```python
from build123d import *

# Parameters (mm, degrees)
SKETCH_1_W                = 42
SKETCH_1_H                = 42
SKETCH_1_R                = 1.85
EXTRUDE_1_DEPTH           = 8
FILLET_2_R                = 2
FILLET_3_R                = 2
FILLET_4_R                = 2
FILLET_5_R                = 2
SKETCH_2_W                = 6
SKETCH_2_H                = 10.5
SKETCH_2_W_2              = 4
SKETCH_2_H_2              = 26
SKETCH_2_W_3              = 13
SKETCH_2_H_3              = 5.5
CUT_EXTRUDE_1_DEPTH       = 6
SKETCH_3_W                = 5.557975162
SKETCH_3_H                = 9
CUT_EXTRUDE_2_DEPTH       = 3
CUT_EXTRUDE_3_DEPTH       = 31.757112998
CUT_EXTRUDE_13_DEPTH      = 31.757112998
SKETCH_6_W                = 14
SKETCH_6_H                = 11
CUT_EXTRUDE_4_DEPTH       = 31.757112998
CUT_EXTRUDE_5_DEPTH       = 3
HOLE_WIZARD_2_D           = 3.6
HOLE_WIZARD_2_DEPTH       = 8
HOLE_WIZARD_2_CSINK_D     = 6.6
HOLE_WIZARD_2_CSINK_ANGLE = 90


with BuildPart() as part:
    # 草图1 → 凸台-拉伸1 (new body)
    with BuildSketch(Plane(origin=(0, 0, 0), x_dir=(1, 0, 0), z_dir=(0, 1, 0))):
        Rectangle(SKETCH_1_W, SKETCH_1_H)
        with Locations(Location((15.5, 15.5, 0), (0, 0, 270))):
            Circle(SKETCH_1_R, mode=Mode.SUBTRACT)
        with Locations(Location((-15.5, 15.5, 0), (0, 0, 270))):
            Circle(SKETCH_1_R, mode=Mode.SUBTRACT)
        with Locations(Location((-15.5, -15.5, 0), (0, 0, 270))):
            Circle(SKETCH_1_R, mode=Mode.SUBTRACT)
        with Locations(Location((15.5, -15.5, 0), (0, 0, 270))):
            Circle(SKETCH_1_R, mode=Mode.SUBTRACT)
    extrude(amount=EXTRUDE_1_DEPTH)

    # 圆角2
    fillet_2_edges = [part.edges().sort_by_distance(p)[0] for p in [
        (-21, 4, -21),
    ]]
    fillet(fillet_2_edges, radius=FILLET_2_R)

    # 圆角3
    fillet_3_edges = [part.edges().sort_by_distance(p)[0] for p in [
        (-21, 4, 21),
    ]]
    fillet(fillet_3_edges, radius=FILLET_3_R)

    # 圆角4
    fillet_4_edges = [part.edges().sort_by_distance(p)[0] for p in [
        (21, 4, 21),
    ]]
    fillet(fillet_4_edges, radius=FILLET_4_R)

    # 圆角5
    fillet_5_edges = [part.edges().sort_by_distance(p)[0] for p in [
        (21, 4, -21),
    ]]
    fillet(fillet_5_edges, radius=FILLET_5_R)

    # 草图2 → 切除-拉伸1 (cut)
    with BuildSketch(Plane.XZ):
        with Locations((18, 7.7)):
            Rectangle(SKETCH_2_W, SKETCH_2_H)
        with Locations((-19, -0.23)):
            Rectangle(SKETCH_2_W_2, SKETCH_2_H_2)
        with Locations((14.5, -9.635)):
            Rectangle(SKETCH_2_W_3, SKETCH_2_H_3)
    extrude(amount=-CUT_EXTRUDE_1_DEPTH, mode=Mode.SUBTRACT)

    # 草图3 → 切除-拉伸2 (cut)
    with BuildSketch(Plane.XZ):
        with Locations((18.221012419, -3)):
            Rectangle(SKETCH_3_W, SKETCH_3_H)
    extrude(amount=-CUT_EXTRUDE_2_DEPTH, mode=Mode.SUBTRACT)

    # 草图5 → 切除-拉伸3 (cut, through all)
    with BuildSketch(Plane.XZ):
        Polygon((-15.5, -21), (-10, -15.5), (10, -15.5), (15.5, -21), align=None)
    extrude(amount=-CUT_EXTRUDE_3_DEPTH, mode=Mode.SUBTRACT)

    # 草图10 → 切除-拉伸13 (cut, through all)
    with BuildSketch(Plane(origin=(0, 8, 0), x_dir=(1, 0, 0), z_dir=(0, 1, 0))):
        with BuildLine():
            Line((7, -21.5), (2.5, -21.5))
            Line((2.5, -21.5), (2.5, -17))
            ThreePointArc((2.5, -17), (10.181980515, -13.818019485), (7, -21.5))
        make_face()
    extrude(amount=-CUT_EXTRUDE_13_DEPTH, mode=Mode.SUBTRACT)

    # 草图6 → 切除-拉伸4 (cut, through all)
    with BuildSketch(Plane.XZ):
        with Locations((-3, 15.5)):
            Rectangle(SKETCH_6_W, SKETCH_6_H)
    extrude(amount=-CUT_EXTRUDE_4_DEPTH, mode=Mode.SUBTRACT)

    # 草图7 → 切除-拉伸5 (cut)
    with BuildSketch(Plane.XZ):
        Polygon((-9.016278831, 15.5), (-15.5, 9.016278831), (-15.5, -9.016278831), (-9.016278831, -15.5), (9.016278831, -15.5), (15.5, -9.016278831), (15.5, 9.016278831), (9.016278831, 15.5), align=None)
    extrude(amount=-CUT_EXTRUDE_5_DEPTH, mode=Mode.SUBTRACT)

    # 打孔尺寸(%根据十字)槽半沉头木螺钉的类型2
    with Locations(Plane(origin=(0, 8, 0), x_dir=(1, 0, 0), z_dir=(0, 1, 0))):
        with Locations((15.5, -15.5), (-15.5, -15.5), (-15.5, 15.5), (15.5, 15.5)):
            CounterSinkHole(HOLE_WIZARD_2_D / 2, HOLE_WIZARD_2_CSINK_D / 2, depth=HOLE_WIZARD_2_DEPTH, counter_sink_angle=HOLE_WIZARD_2_CSINK_ANGLE)


solid = part.part
```
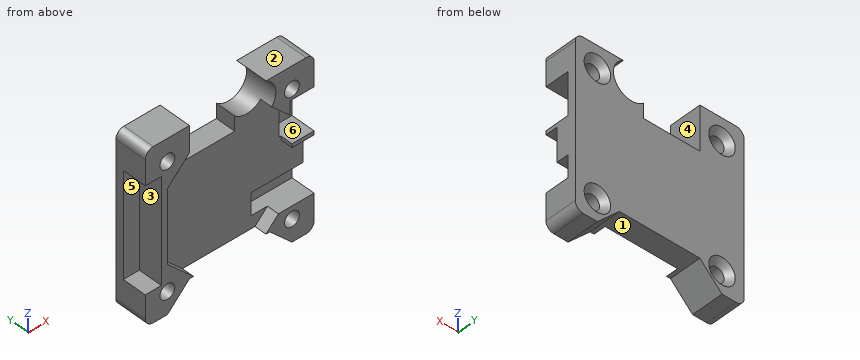
Design review of the part built by this model. Coordinates are the model's own, in mm. Face numbers are marked on the shaded views. A direction names the side the tool comes from. Round coordinates to 2 decimals unless told otherwise and drop trailing zeros. Write each loop counter-clockwise with the first axis right and the second up, starting at its lowest first coordinate (ties: lowest second). Pieces come first, ordered by that corner, then holes. Notation, with made-up numbers: (51.5, 39.25) -> (95.5, 39.25) arc R23 cw to (95.5, 67.25) -> close; hole circle Ø10 at (19.5, 76). An arc over 180 degrees is marked (long way). Answer in a Markdown table with one row per item.
Q1. For the marked faces 4, 5 and 6, list the 3-axis set-ups (+Z, -Z, +X, -X, +Y, -Y) from which the entire face can be reached by the end or side of a thin tool; tool diameter is ignored.
The answers:
| item | result |
|---|---|
| face 4 | +Z, +Y, -Y |
| face 5 | -X, -Y |
| face 6 | +X, -Y |
Q2. Clearance check with flat-ended pins moving along their axes: pin 1 Ø0.8 at (y, z) = (2, 2) entering from -X; pin 2 Ø9 at (x, z) = (-5, 4.5) entering from -Y; pin 3 Ø3.5 at (x, y) = (13, 4) entering from -Z. State where each tip first meets the part, or that it passes through.
The answers:
| item | result |
|---|---|
| pin 1 | x = -17 |
| pin 2 | y = 3 |
| pin 3 | z = -20.25 |
Q3. Take a section at B-B, the plane z = 0. State the section outline as (x, y) points.
The answers:
| item | result |
|---|---|
| outline | (-21, 6) -> (-17, 6) -> (-17, 0) -> (-15.5, 0) -> (-15.5, 3) -> (21, 3) -> (21, 8) -> (-21, 8) -> close |
Q4. Draft analysis for pull direction X (two halves, no side actions). For the marked faces 1, 2 and 3, state which applies: +X half, -X half, draft (parallel to the pull), parting line (faces both ways), or undercut.
The answers:
| item | result |
|---|---|
| face 1 | undercut |
| face 2 | draft |
| face 3 | -X half |
Q5. To check wall thickness, follow L1, parallel to Z at x = 16.5, y = 2 (3 decimals); L2, parallel to Z at x = 10.5, y = 1.25; L3, parallel to X at y = 2.5, z = 15.5. State the ranges of each line that lie inside material, in increasing order. Write a range as [from, to].
The answers:
| item | result |
|---|---|
| L1 | [-21, -17.056], [-13.944, -12.385], [1.5, 2.45], [12.95, 13.944], [17.056, 21] |
| L2 | [-16, -14.02], [14.02, 14.17], [19.83, 21] |
| L3 | [-21, -17.35], [-13.65, -10], [11.24, 13.65], [17.35, 21] |
Q6. Take a section at A-A, the plane y = 2.25. Count the separate pieces of the cut face and the enclosed holes in it, then the cut area to 3 significant figures.
The answers:
| item | result |
|---|---|
| separate pieces | 4 |
| enclosed holes | 4 |
| area | 337 mm² |
Q7. Take a section at C-C, the plane x = 7. State the section outline as (y, z) points, then the cut area to 3 significant figures.
The answers:
| item | result |
|---|---|
| outline | (3, -15.5) -> (8, -15.5) -> (8, 12.5) -> (3, 12.5) -> close |
| area | 140 mm² |
Q8. Take a section at D-D, the plane z = 15.5. State the section outline as (x, y) points, then the cut area to 3 significant figures.
The answers:
| item | result |
|---|---|
| outline | (-21, 0) -> (-17.35, 0) -> (-17.35, 6.55) -> (-18.8, 8) -> (-21, 8) -> close; (-13.65, 0) -> (-10, 0) -> (-10, 8) -> (-12.2, 8) -> (-13.65, 6.55) -> close; (11.24, 0) -> (13.65, 0) -> (13.65, 6.55) -> (12.2, 8) -> (11.24, 8) -> close; (17.35, 0) -> (21, 0) -> (21, 8) -> (18.8, 8) -> (17.35, 6.55) -> close |
| area | 103 mm² |
